The figure shows three views and two pictorial views of one solid part (mm, origin at its lowest corner). Answer the questions. A direction names the side the tool comes from. Coordinates: 2 decimals unless noted, no trailing zeros. Write each loop counter-clockwise with the first axis right and the second up, starting at its lowest first coordinate (ties: lowest second). Pieces come first, ordered by that corner, then holes.
Item 1: A tool of negligible diameter and unlimited length cuts with its end or side. For the marked faces 1, 2 and 3, from which of +Z, -Z, +X, -X, +Y, -Y can it reach the whole face along a straight path? Write none if from no direction.
Item 2: Each of these flat-tipped pins is pushed along its axis until it touches: P1, Ø5, axis at x = 6.35, y = 63.5, coming from the +Z side; P2, Ø4, axis at x = 19, z = 9.5, coming from the +Y side; P3, Ø20.5, axis at x = 21.5, y = 6.5, coming from the -Z side; P4, Ø10, axis at x = 19, z = 9, coming from the -Y side. Where does it stop, or does it pass through?
Item 3: Straight lines are drawn through the part: probe 1 along Z at (x, y) = (24, 62); probe 2 along Z at (x, y) = (19.5, 24.5). For each, find the intervals that lie inside material, in ascending order.
Item 4: Determine the mould class of the marked faces 4, 5, 6 and 7 for opening direction Z: released by +Z, released by -Z, zero draft, split by the parting line, or undercut.
Item 5: Section C-C (x = 29) is taken. Give the vertices of the cut face in (y, z), then the cut area to 3 significant figures.
Item 6: Section D-D (z = 29.5) is taken. Give the vertices of the cut face in (x, y) (3 decimals), then the cut area to 3 significant figures.
Item 7: Section B-B (y = 43.5) is taken. Give the vertices of the cut face in (x, z), then the cut area to 3 significant figures.
Item 8: Section A-A (y = 63.5) is taken. Give the vertices of the cut face in (x, z) (3 decimals), then the cut area to 3 significant figures.
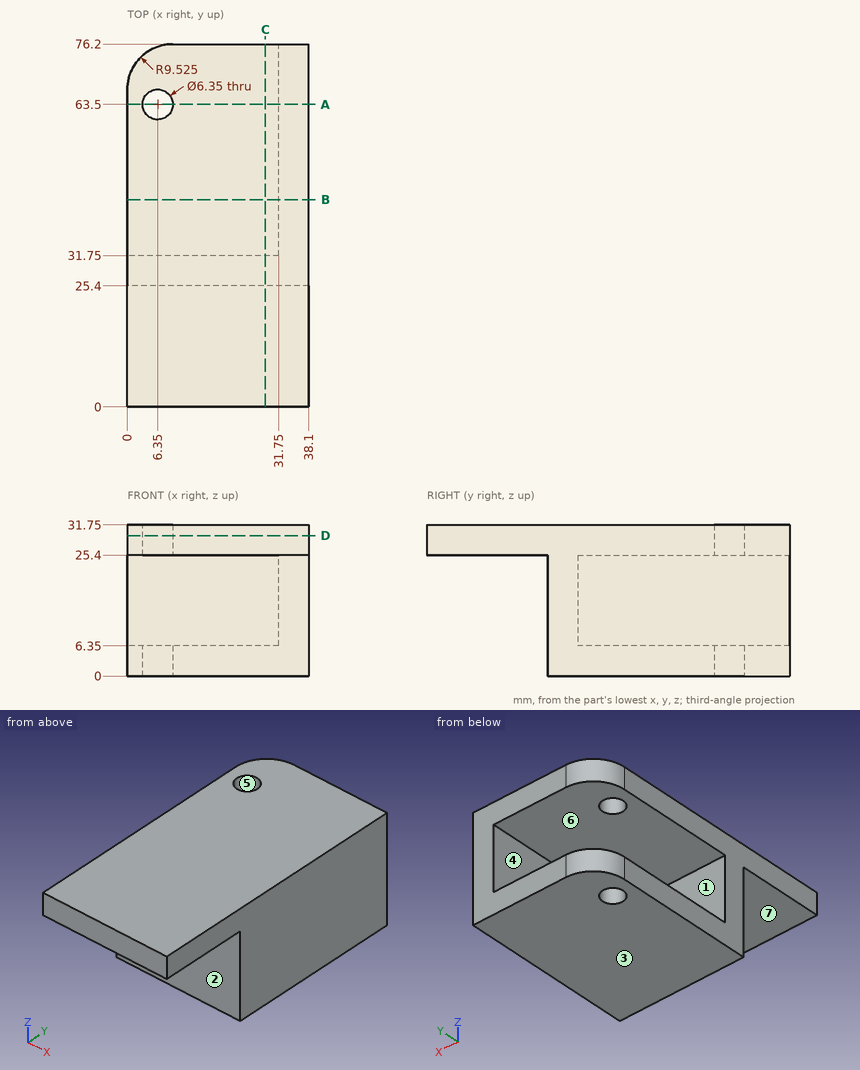
Established:
1. face 1: -X, +Y
1. face 2: -Z, +X, -X, -Y
1. face 3: -Z, +X, -X, +Y, -Y
2. P1: passes through
2. P2: stops at y = 31.75
2. P3: stops at z = 25.4
2. P4: stops at y = 25.4
3. probe 1: z = 0 to 6.35, 25.4 to 31.75
3. probe 2: z = 25.4 to 31.75
4. face 4: undercut
4. face 5: zero draft
4. face 6: undercut
4. face 7: released by -Z
5. outline: (0, 25.4) - (25.4, 25.4) - (25.4, 0) - (76.2, 0) - (76.2, 6.35) - (31.75, 6.35) - (31.75, 25.4) - (76.2, 25.4) - (76.2, 31.75) - (0, 31.75) - close
5. area: 927 mm2
6. outline: (0, 0) - (38.1, 0) - (38.1, 76.2) - (9.525, 76.2) arc R9.525 ccw to (0, 66.675) - close; hole circle Ø6.35 at (6.35, 63.5)
6. area: 2,850 mm2
7. outline: (0, 0) - (38.1, 0) - (38.1, 31.75) - (0, 31.75) - (0, 25.4) - (31.75, 25.4) - (31.75, 6.35) - (0, 6.35) - close
7. area: 605 mm2
8. outline: (0, 0) - (3.175, 0) - (3.175, 6.35) - (0, 6.35) - close; (0, 25.4) - (3.175, 25.4) - (3.175, 31.75) - (0, 31.75) - close; (9.525, 0) - (38.1, 0) - (38.1, 31.75) - (9.525, 31.75) - (9.525, 25.4) - (31.75, 25.4) - (31.75, 6.35) - (9.525, 6.35) - close
8. area: 524 mm2
